Read the model definition and answer for the solid it produces. Units are mm, in the model's axes. Give positions to 0.01 mm unless a question says otherwise; leave off trailing zeros. Order: outer loops, then holes, each group sorted by start corner. A loop starts at its lowest first (then second) coordinate and runs counter-clockwise, first axis right, second up.
Item 1: A cutting plane is placed at A-A (z = 0.4). Write down the section's boundary in (x, y).
Item 2: A cutting plane is placed at C-C (x = 35). Write down the section's boundary in (y, z).
Item 3: The mould has two halves that part along X. Classify faces 1 (the face through (35.724, 25.441, 0.493)), 2 (the face through (-35.724, 25.441, 0.493)), 3 (the face through (0, 13, 0)): +X half, -X half, draft (parallel to the pull), parting line (faces both ways), or undercut.
Item 4: A cutting plane is placed at B-B (y = 21). Write down the section's boundary in (x, z).
Item 5: A cutting plane is placed at D-D (x = 5.5). Write down the section's boundary in (y, z), plus the area to 3 significant figures.
Item 6: Find the intervals of material crossed by line 1 along X through (y, z) = (20.25, 0.9); line 2 along X through (y, z) = (20.5, 0.25); line 3 along Y through (x, z) = (35.5, 0.8), in increasing order.
from build123d import *

# Parameters (mm, degrees)
PAD_DEPTH = 1


with BuildPart() as clone_of_countersunk001:
    # Sketch007 → Revolution001 (revolve)
    with BuildSketch(Plane.YZ):
        Polygon((3.2, 0), (1.5, -1.7), (1.5, -15), (0, -15), (0, 0), align=None)
    revolve(axis=Axis((0, 0, 0), (0, 0, 1)))


with BuildPart() as clone_of_countersunk001_1:
    # Clone placement: moved
    add(clone_of_countersunk001.part.moved(Location((35, 21, 1))))


with BuildPart() as countersunkcut:
    # Sketch → Pad (new body)
    with BuildSketch(Plane.XY):
        with BuildLine():
            ThreePointArc((35.990539, 16.610372), (35.549071, 25.466377), (32.975752, 16.980993))
            ThreePointArc((0, 13.6), (16.574312, 14.447458), (32.975752, 16.980993))
            Line((0, 13.6), (0, 12.6))
            ThreePointArc((0, 12.6), (18.106642, 13.605686), (35.990539, 16.610372))
        make_face()
    extrude(amount=PAD_DEPTH)

    # Cut: cut Clone of Countersunk001
    add(clone_of_countersunk001_1.part, mode=Mode.SUBTRACT)


with BuildPart() as part_mirroring:
    # Part__Mirroring: instance of CountersunkCut
    add(countersunkcut.part.mirror(Plane(origin=(0, 0, 0), x_dir=(0, -1, 0), z_dir=(1, 0, 0))))


with BuildPart() as sidemirror:
    # Fusion base: copy of CountersunkCut
    add(countersunkcut.part)

    # Fusion: union Part__Mirroring
    add(part_mirroring.part)


solid = sidemirror.part
Response values:
1. outline: (-35.99, 16.61) arc R163.5 ccw to (0, 12.6) arc R163.5 ccw to (35.99, 16.61) arc R4.5 ccw (long way) to (32.98, 16.98) arc R162.5 cw to (-32.98, 16.98) arc R4.5 ccw (long way) to start; hole circle Ø5.2 at (-35, 21); hole circle Ø5.2 at (35, 21)
2. outline: (16.39, 0) - (18.8, 0) - (17.8, 1) - (16.39, 1) - close; (23.2, 0) - (25.5, 0) - (25.5, 1) - (24.2, 1) - close
3. face 1: undercut
3. face 2: undercut
3. face 3: draft
4. outline: (-39.5, 0) - (-37.2, 0) - (-38.2, 1) - (-39.5, 1) - close; (-32.8, 0) - (-30.5, 0) - (-30.5, 1) - (-31.8, 1) - close; (30.5, 0) - (32.8, 0) - (31.8, 1) - (30.5, 1) - close; (37.2, 0) - (39.5, 0) - (39.5, 1) - (38.2, 1) - close
5. outline: (12.69, 0) - (13.69, 0) - (13.69, 1) - (12.69, 1) - close
5. area: 1.00 mm2
6. line 1: x = -39.44 to -38.01, -31.99 to -30.56, 30.56 to 31.99, 38.01 to 39.44
6. line 2: x = -39.47 to -37.4, -32.6 to -30.53, 30.53 to 32.6, 37.4 to 39.47
6. line 3: y = 16.5 to 18.04, 23.96 to 25.47
